Geometry: final body of the model. Coordinates: model frame, mm. A direction names the side the tool comes from. Give positions to 0.01 mm unless a question says otherwise; leave off trailing zeros. Loops run counter-clockwise (first coordinate to the right, second up) from the corner with the lowest first, then second, coordinate; pieces in that order, holes last. Notation, with made-up numbers: (83, 69.5) -> (113, 69.5) arc R19 ccw to (113, 103.5) -> close; hole circle Ø6 at (-33.75, 61). An arc over 180 degrees is marked (long way). One line per item, written item: value. Start each with the question number.
Autodesk Inventor part; units mm, degrees
ref_plane "YZ Plane" through (0, 0, 0) normal (1, 0, 0) x (0, 1, 0)
ref_plane "XZ Plane" through (0, 0, 0) normal (0, 1, 0) x (-1, 0, 0)
ref_plane "XY Plane" through (0, 0, 0) normal (0, 0, 1) x (1, 0, 0)
sketch "Skizze1" plane through (0, 0, 0) normal (0, 1, 0) x (-1, 0, 0)
  arc A0 (5, 0) -> (-5, 0) centre (0, 0) ccw
  circle A1 centre (0, 0) radius 1.8
  line L0 (-5, 0) -> (-5, -29.2)
  line L1 (-5, -29.2) -> (0.5, -29.2)
  line L2 (5, 0) -> (5, -12)
  line L3 (5, -12) -> (0.5, -29.2)
  dimension "d0" = 10
  dimension "d1" = 3.6
  dimension "d2" = 29.2
  dimension "d3" = 5.5
  dimension "d4" = 12
extrude "Extrusion1" add sketch "Skizze1" along normal blind 1.5
sketch "Skizze2" plane through (0, 1.5, 0) normal (0, 1, 0) x (1, 0, 0)
  line L0 (4.9805, 29.2565) -> (5, 6.2565)
  line L1 (5, 0) -> (5, 29.2)
  line L2 (5, 29.2) -> (2, 29.2)
  line L3 (2, 29.2) -> (2, 10.7)
  line L4 (2, 10.7) -> (5, 6.2565)
  point P0 (0, 0)
  dimension "d7" = 23
  dimension "d8" = 3
  dimension "d9" = 18.5
extrude "Extrusion2" add sketch "Skizze2" along normal blind 4.4
sketch "Skizze3" plane through (2, 1.5, -29.2) normal (-1, 0, 0) x (0, 0, 1)
  line L0 (22.9435, 4.4) -> (0, 4.4) construction
  line L1 (0, 4.4) -> (3.5, 4.4) construction
  line L2 (0, 3.6562) -> (11.2, 3.6562) construction
  line L3 (3.5, 4.4) -> (7.8, 4.4) construction
  line L4 (11.2, 4.4) -> (15.5, 4.4) construction
  line L5 (3.5, 4.4) -> (7.8, 4.4) construction
  line L6 (5.15, 2.75) -> (6.15, 2.75)
  arc A0 (3.5, 4.4) -> (5.15, 2.75) centre (5.15, 4.4) ccw
  arc A1 (6.15, 2.75) -> (7.8, 4.4) centre (6.15, 4.4) ccw
  line L7 (11.2, 4.4) -> (15.5, 4.4) construction
  line L8 (12.85, 2.75) -> (13.85, 2.75)
  arc A2 (11.2, 4.4) -> (12.85, 2.75) centre (12.85, 4.4) ccw
  arc A3 (13.85, 2.75) -> (15.5, 4.4) centre (13.85, 4.4) ccw
  line L9 (3.5, 4.4) -> (7.8, 4.4)
  line L10 (11.2, 4.4) -> (15.5, 4.4)
  point P0 (29.2, -1.5)
  point P1 (5.65, 4.4)
  point P2 (13.35, 4.4)
extrude "Extrusion3" cut sketch "Skizze3" against normal blind 4.4
fillet "Rundung1" radius 1.5 6 edges at (2, 4.25, -23.55) (2, 4.7333, -25.2167) (2, 4.7333, -21.8833) (2, 4.7333, -17.5167) (2, 4.7333, -14.1833) (2, 4.25, -15.85)
mirror "Spiegeln1" about plane through (3.6338, 5.9, -18.2488) normal (0, 1, 0)
properties part number "chain_end_elmt"
Item 1: Section A-A, the plane z = -3. Output: boundary loops of the cut face in (x, y), then the cut area to 3 significant figures.
Item 2: Section D-D, the plane x = -3.5. Output: boundary loops of the cut face in (y, z), then the cut area to 3 significant figures.
Item 3: Access query for faces 1 (the face through (4.2, 7.55, -23.5)), 2 (the face through (0, 10.3, -8)), 3 (the face through (2.45, 3.82, -15.84)). Directions: +Z, -Z, +X, -X, +Y, -Y. A direction counts if a zero-diameter tool reaches every point of the face in a straight line with its end or side. Return the directions, or none.
Item 4: Ray query, line 1 along Y through (x, z) = (-0.25, -19); line 2 along Z through (x, y) = (0, 1.1); line 3 along X through (y, z) = (6.25, -10). Return the intervals inside material, ascending. Write a range as [from, to].
Item 5: Pin query (flat end, axial travel): pin 1 (2 mm diameter, centred on x = 0, z = 0, fed in from +Y). Return the tip coordinate at first contact, or that it passes through.
Item 6: Section B-B, the plane x = 0. Output: boundary loops of the cut face in (y, z), then the cut area to 3 significant figures.
Item 7: Mould query, pull axis Z, two halves, no side actions, for faces 4 (the face through (-5, 1, -6)), 5 (the face through (-2.78, 0.74, -20.48)), 6 (the face through (4.2, 5.9, -21.4)), 7 (the face through (3.48, 5.84, -8.51)). Classes: pulls with the +Z half, pulls with the -Z half, needs draft (parallel to the pull), parting line crosses it, or undercut.
Item 8: Section C-C, the plane y = 11. Output: boundary loops of the cut face in (x, z), then the cut area to 3 significant figures.
Geometry check:
1. outline: (-5, 0) -> (5, 0) -> (5, 1.5) -> (-5, 1.5) -> close; (-5, 10.3) -> (5, 10.3) -> (5, 11.8) -> (-5, 11.8) -> close
1. area: 30.0 mm2
2. outline: (0, -17.73) -> (1.5, -17.73) -> (1.5, 3.57) -> (0, 3.57) -> close; (10.3, -17.73) -> (11.8, -17.73) -> (11.8, 3.57) -> (10.3, 3.57) -> close
2. area: 63.9 mm2
3. face 1: +X, -X
3. face 2: +Z, -X
3. face 3: -X
4. line 1: y = [0, 1.5], [10.3, 11.8]
4. line 2: z = [-29.2, -1.8], [1.8, 5]
4. line 3: x = [2.47, 5]
5. pin 1: passes through
6. outline: (0, -29.2) -> (1.5, -29.2) -> (1.5, -1.8) -> (0, -1.8) -> close; (0, 1.8) -> (1.5, 1.8) -> (1.5, 5) -> (0, 5) -> close; (10.3, -29.2) -> (11.8, -29.2) -> (11.8, -1.8) -> (10.3, -1.8) -> close; (10.3, 1.8) -> (11.8, 1.8) -> (11.8, 5) -> (10.3, 5) -> close
6. area: 91.8 mm2
7. face 4: needs draft
7. face 5: pulls with the -Z half
7. face 6: undercut
7. face 7: pulls with the +Z half
8. outline: (-5, -12) -> (-0.5, -29.2) -> (5, -29.2) -> (5, 0) arc R5 ccw to (-5, 0) -> close; hole circle Ø3.6 at (0, 0)
8. area: 282 mm2
